Build history of the part. All positions in model axes, mm. Face numbers are marked on the shaded views. A direction names the side the tool comes from. Give positions to 0.01 mm unless a question says otherwise; leave off trailing zeros. Write each loop counter-clockwise with the first axis right and the second up, starting at its lowest first coordinate (ties: lowest second). Pieces come first, ordered by that corner, then holes.
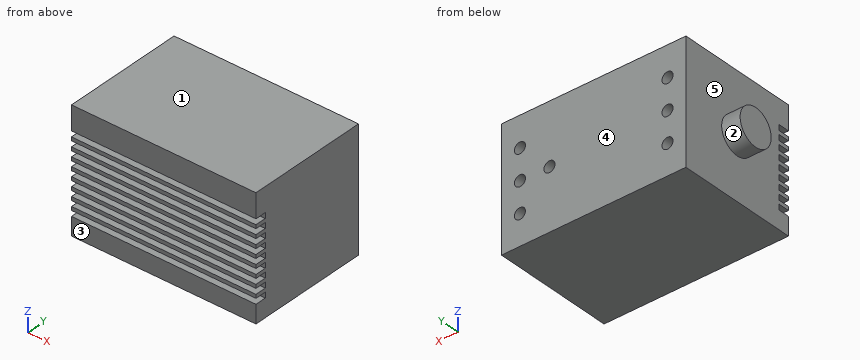
from build123d import *

# Parameters (mm, degrees)
F0_W     = 50
F0_H     = 33
F1_DEPTH = 33
F2_W     = 6
F2_H     = 1.5
F3_DEPTH = 50.001
F4_R     = 5
F5_DEPTH = 5
F6_R     = 1.5
F7_DEPTH = 7


with BuildPart() as f1:
    # F0 (on Top) → F1 (new body)
    with BuildSketch(Plane.XY):
        Rectangle(F0_W, F0_H)
    extrude(amount=F1_DEPTH)

    # F2 (on face) → F3 (cut, through all)
    with BuildSketch(Plane.YZ.offset(25)):
        with Locations((-16.5, 25.702117)):
            Rectangle(F2_W, F2_H)
        with Locations((-16.5, 23.202117)):
            Rectangle(F2_W, F2_H)
        with Locations((-16.5, 20.702117)):
            Rectangle(F2_W, F2_H)
        with Locations((-16.5, 18.202117)):
            Rectangle(F2_W, F2_H)
        with Locations((-16.5, 15.702117)):
            Rectangle(F2_W, F2_H)
        with Locations((-16.5, 13.202117)):
            Rectangle(F2_W, F2_H)
        with Locations((-16.5, 10.702117)):
            Rectangle(F2_W, F2_H)
        with Locations((-16.5, 8.202117)):
            Rectangle(F2_W, F2_H)
        with Locations((-16.5, 5.702117)):
            Rectangle(F2_W, F2_H)
    extrude(amount=-F3_DEPTH, mode=Mode.SUBTRACT)

    # F4 (on face) → F5 (join)
    with BuildSketch(Plane(origin=(-25, 0, 0), x_dir=(0, -1, 0), z_dir=(-1, 0, 0))):
        with Locations((0, 16.5)):
            Circle(F4_R)
    extrude(amount=F5_DEPTH)

    # F6 (on face) → F7 (cut)
    with BuildSketch(Plane(origin=(0, 16.5, 0), x_dir=(-1, 0, 0), z_dir=(0, 1, 0))):
        with Locations((-20, 8.25)):
            Circle(F6_R)
        with Locations((-20, 16.5)):
            Circle(F6_R)
        with Locations((-20, 24.75)):
            Circle(F6_R)
        with Locations((-12, 16.5)):
            Circle(F6_R)
        with Locations((20, 16.5)):
            Circle(F6_R)
        with Locations((20, 8.25)):
            Circle(F6_R)
        with Locations((20, 24.75)):
            Circle(F6_R)
    extrude(amount=-F7_DEPTH, mode=Mode.SUBTRACT)


solid = f1.part
(1) Saw through at D-D, the plane z = 27.5. List the corners of the cut face in (x, y).
(2) Drop flat-ended pins along their axis: pin 1 (0.8 mm diameter, centred on x = 5, z = 10.5, fed in from -Y); pin 2 (2 mm diameter, centred on y = -3.5, z = 9.5, fed in from -X). Give the stop position or say it passes through.
(3) Saw through at C-C, the plane x = -26. List the corners of the cut face in (y, z).
(4) Probe line 1 (Z direction, x = 20, y = 12); line 2 (Z direction, x = 12, y = 13); line 3 (X direction, y = 14, z = 16). List the from-to ranges inside material, lowest first.
(5) 3-axis set-ups, long thin cutter, end or side, ignore diameter. For the marked faces 4 and 5: which of +Z, -Z, +X, -X, +Y, -Y reach the whole face in a straight line?
(6) Saw through at B-B, the plane y = 2.5. List the corners of the cut face in (x, z), plus the area to 3 significant figures.
(7) Mould opens along Y. For the marked faces 1, 2 and 3 say: +Y half, -Y half, draft (parallel to the pull), parting line (faces both ways), or undercut.
(8) Saw through at A-A, the plane z = 8.25. List the corners of the cut face in (x, y), plus the area to 3 significant figures.
Computed values:
1. outline: (-25, -16.5) - (25, -16.5) - (25, 16.5) - (-25, 16.5) - close
2. pin 1: stops at y = -13.5
2. pin 2: stops at x = -25
3. outline: circle Ø10 at (0, 16.5)
4. line 1: z = 0 to 6.75, 9.75 to 15, 18 to 23.25, 26.25 to 33
4. line 2: z = 0 to 15, 18 to 33
4. line 3: x = -25 to -21.41, -18.59 to 10.59, 13.41 to 18.59, 21.41 to 25
5. face 4: +Z, -Z, +X, -X, +Y
5. face 5: -X
6. outline: (-30, 12.17) - (-25, 12.17) - (-25, 0) - (25, 0) - (25, 33) - (-25, 33) - (-25, 20.83) - (-30, 20.83) - close
6. area: 1,690 mm2
7. face 1: draft
7. face 2: parting line
7. face 3: -Y half
8. outline: (-25, -13.5) - (25, -13.5) - (25, 16.5) - (21.5, 16.5) - (21.5, 9.5) - (18.5, 9.5) - (18.5, 16.5) - (-18.5, 16.5) - (-18.5, 9.5) - (-21.5, 9.5) - (-21.5, 16.5) - (-25, 16.5) - close
8. area: 1,460 mm2
